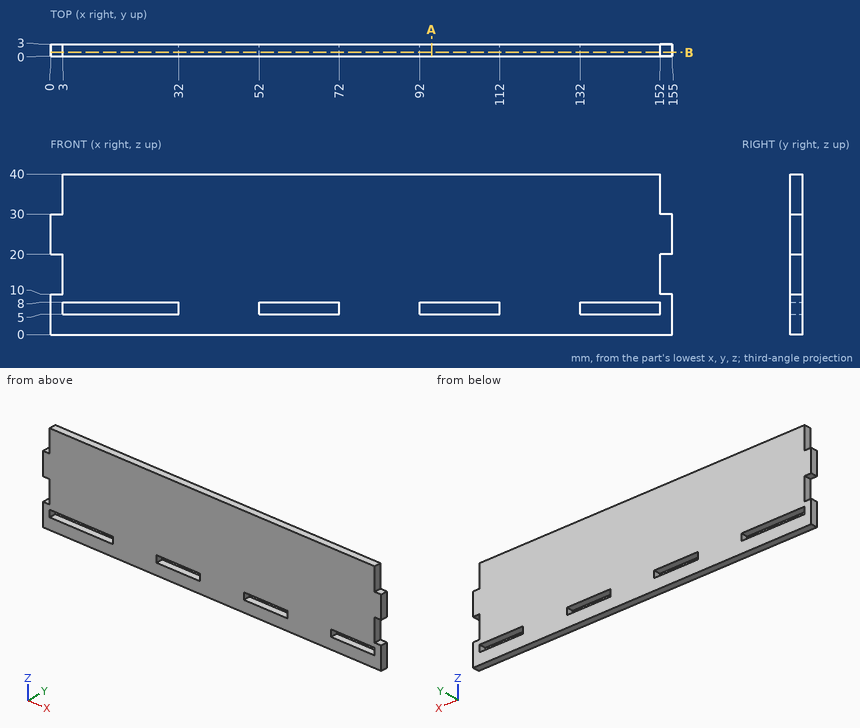
Drawing for the job (mm, zero at the part's lowest x, y, z). Coordinates: 2 decimals unless noted, no trailing zeros. Order: outer loops, then holes, each group sorted by start corner. A loop starts at its lowest first (then second) coordinate and runs counter-clockwise, first axis right, second up. Notation, with made-up numbers: (-4.5, 50.25) - (1.5, 50.25) arc R7 ccw to (1.5, 60.25) - close; hole circle Ø3 at (-19.5, 18.25). An arc over 180 degrees is marked (long way). Use a Markdown table: item, result. Add a question column.
(1) Flat gauge pins, fed straight in: pin 1 (1.5 mm diameter, centred on y = 2, z = 15, fed in from -X); pin 2 (0.9 mm diameter, centred on x = 102.5, y = 2, fed in from -Z). Where does each tip first touch, or does it go through?
(2) Saw through at A-A (x = 95). Give the cut face in (y, z).
(3) Drill centre lines: line 1 along X through (y, z) = (2.6, 6); line 2 along Z through (x, y) = (56, 1.3); line 3 along X through (y, z) = (0.4, 13). Where is each one in solid material? Low to high. Write a range as [from, to].
(4) Saw through at B-B (y = 0.9). Count the separate pieces of the cut face and the enclosed holes in it, then the cut area to 3 significant figures.
Solved:
| question | item | result |
|---|---|---|
| 1 | pin 1 | stops at x = 3 |
| 1 | pin 2 | stops at z = 0 |
| 2 | outline | (0, 0) - (3, 0) - (3, 5) - (0, 5) - close; (0, 8) - (3, 8) - (3, 40) - (0, 40) - close |
| 3 | line 1 | x = [0, 3], [32, 52], [72, 92], [112, 132], [152, 155] |
| 3 | line 2 | z = [0, 5], [8, 40] |
| 3 | line 3 | x = [3, 152] |
| 4 | separate pieces | 1 |
| 4 | enclosed holes | 4 |
| 4 | area | 5,810 mm² |
